Autodesk Inventor part; units mm, degrees
ref_plane "YZ Plane" through (0, 0, 0) normal (1, 0, 0) x (0, 1, 0)
ref_plane "XZ Plane" through (0, 0, 0) normal (0, 1, 0) x (-1, 0, 0)
ref_plane "XY Plane" through (0, 0, 0) normal (0, 0, 1) x (1, 0, 0)
sketch "Sketch1" plane through (0, 0, 0) normal (1, 0, 0) x (0, 1, 0)
  line L0 (0, 0) -> (-10, 0)
  line L1 (-10, 0) -> (-10, 10)
  line L2 (-10, 10) -> (0, 10)
  line L3 (0, 10) -> (0, 0)
  line L4 (-9, 9) -> (0, 9)
  line L5 (0, 9) -> (0, 0)
  line L6 (0, 0) -> (-9, 0)
  line L7 (-9, 0) -> (-9, 9)
  dimension "d0" = 10
  dimension "d1" = 1
extrude "Extrusion1" add sketch "Sketch1" along normal blind 11 contours L0 L1 L2 L3 L4 L7
properties part number "CouplerL" material "Stainless Steel"
Verification items for the finished model (mm, model axes). A direction names the side the tool comes from. Give positions to 0.01 mm unless a question says otherwise; leave off trailing zeros. Write each loop counter-clockwise with the first axis right and the second up, starting at its lowest first coordinate (ties: lowest second). Pieces come first, ordered by that corner, then holes. Notation, with made-up numbers: (70.5, 14.25) - (122.5, 14.25) arc R20 cw to (122.5, 27.25) - close; hole circle Ø2 at (60, 72.5). An arc over 180 degrees is marked (long way). Answer as CSV lines item,"result". Start each with the question number.
1. Sectioned sample at A-A (z = 5.75). Record the boundary of the cut face in (x, y), then the cut area to 3 significant figures.
2. Sectioned sample at B-B (x = 10). Record the boundary of the cut face in (y, z).
3. Depth check by flat-ended pin: pin 1 (4 mm diameter, centred on y = -5.5, z = 6, fed in from -X) (3 decimals); pin 2 (1.5 mm diameter, centred on x = 5.5, y = -6, fed in from -Z); pin 3 (1.5 mm diameter, centred on x = 9, z = 6.5, fed in from +Y); pin 4 (4 mm diameter, centred on y = -3.5, z = 8, fed in from -X). Enter the tip coordinate at first touch or a pass-through.
4. Thickness scan on line 1 (Y direction, x = 5.75, z = 7.75); line 2 (Z direction, x = 1.75, y = -7). Record the ranges inside material, lowest first.
5. Sectioned sample at C-C (y = -8). Record the boundary of the cut face in (x, z), then the cut area to 3 significant figures.
6. Set-up check for faces 1 (the face through (5, -5, 9)), 2 (the face through (5, -10, 5)): record each of +Z, -Z, +X, -X, +Y, -Y from which the full face is reachable in a straight line by a thin tool's end or side.
Derived:
1,outline,"(0, -10) - (11, -10) - (11, -9) - (0, -9) - close"
1,area,"11.0 mm²"
2,outline,"(-10, 0) - (-9, 0) - (-9, 9) - (0, 9) - (0, 10) - (-10, 10) - close"
3,pin 1,"through"
3,pin 2,"z = 9"
3,pin 3,"y = -9"
3,pin 4,"x = 0"
4,line 1,"-10 to -9"
4,line 2,"9 to 10"
5,outline,"(0, 9) - (11, 9) - (11, 10) - (0, 10) - close"
5,area,"11.0 mm²"
6,face 1,"-Z, +X, -X, +Y"
6,face 2,"+Z, -Z, +X, -X, -Y"
